Work out the finished part from the listing and answer in its coordinate system (mm). A direction names the side the tool comes from. Coordinates: 2 decimals unless noted, no trailing zeros. Order: outer loops, then holes, each group sorted by start corner. A loop starts at its lowest first (then second) coordinate and runs counter-clockwise, first axis right, second up. Notation, with made-up numbers: M 19.25,61.25 L 28.25,61.25 A21 cw 28.25,82.25 Z; hole C -5.75,-17 d3. An arc over 180 degrees is marked long. Answer in a Markdown table with one row per item. Add a question column.
Item 1: The mould has two halves that part along X. Classify faces 1 (the face through (8.5, 0.07, 78.52)), 2 (the face through (-33.89, -24.17, 21.43)), 3 (the face through (-26.45, 31, 12)): released by +X, released by -X, zero draft, split by the parting line, or undercut.
Item 2: Which of the six approach directions +Z, -Z, +X, -X, +Y, -Y give full straight-line access (tool end or side, diameter ignored) to faces 4 (the face through (26.45, -28, 17)), 5 (the face through (-33.9, 24.6, 22)), 6 (the face through (33.9, 24.6, 22))?
Item 3: The part is cut by section C-C (z = 65). Write down the section's boundary in (x, y), then the cut area to 3 significant figures.
Item 4: The part is cut by section B-B (y = 0). Write down the section's boundary in (x, z).
Item 5: Consider line 1 (Y direction, x = -10, z = 79.2); line 2 (X direction, y = -24, z = 46.5); line 3 (Z direction, x = 5.5, y = 17). Determine where each line is inside the solid, lowest interval first. Write a range as from..to.
Item 6: The part is cut by section D-D (y = 19.5). Write down the section's boundary in (x, z), then the cut area to 3 significant figures.
Item 7: A flat-ended cylindrical pin translates along its axis: pin 1 Ø4 at (x, y) = (-10, 25) entering from -Z. Find the tip coordinate at first contact, or state that the pin passes through.
Item 8: The part is cut by section A-A (x = -10). Write down the section's boundary in (y, z), then the cut area to 3 significant figures.
from build123d import *

# Parameters (mm, degrees)
SKETCH_1_W          = 52.9
SKETCH_1_H          = 81.56
EXTRUDE_1_DEPTH     = 80.99
SKETCH_2_W          = 32.9
SKETCH_2_H          = 61.56
CUT_EXTRUDE_1_DEPTH = 75.99
EXTRUDE_2_DEPTH     = 15.1
SKETCH_4_R          = 1.5
CUT_EXTRUDE_2_DEPTH = 100.743626363


with BuildPart() as part:
    # 草图1 → 凸台-拉伸1 (new body)
    with BuildSketch(Plane.XY):
        Rectangle(SKETCH_1_W, SKETCH_1_H)
    extrude(amount=EXTRUDE_1_DEPTH)

    # 草图2 → 切除-拉伸1 (cut)
    with BuildSketch(Plane(origin=(0, 0, 0), x_dir=(-1, 0, 0), z_dir=(0, 0, -1))):
        Rectangle(SKETCH_2_W, SKETCH_2_H)
    extrude(amount=-CUT_EXTRUDE_1_DEPTH, mode=Mode.SUBTRACT)

    # 草图3 → 凸台-拉伸2 (add)
    with BuildSketch(Plane.ZY.offset(26.45)):
        Polygon((80.99, 40.78), (43.47, 40.78), (0, 8.02), (0, -8.02), (43.47, -40.78), (80.99, -40.78), align=None)
    extrude_2 = extrude(amount=EXTRUDE_2_DEPTH)

    # 镜向1: 凸台-拉伸2 across plane
    add(extrude_2.mirror(Plane(origin=(0, 0, 0), x_dir=(0, 0, 1), z_dir=(1, 0, 0))))

    # 草图4 → 切除-拉伸2 (cut, through all)
    with BuildSketch(Plane.XY.offset(80.99)):
        with Locations((-10, 25)):
            Circle(SKETCH_4_R)
        with Locations((10, 25)):
            Circle(SKETCH_4_R)
        with Locations((-10, -25)):
            Circle(SKETCH_4_R)
        with Locations((10, -25)):
            Circle(SKETCH_4_R)
        with Locations((-10, 0)):
            Circle(SKETCH_4_R)
        with Locations((10, 0)):
            Circle(SKETCH_4_R)
    extrude(amount=-CUT_EXTRUDE_2_DEPTH, mode=Mode.SUBTRACT)


solid = part.part
Reply:
| question | item | result |
|---|---|---|
| 1 | face 1 | undercut |
| 1 | face 2 | zero draft |
| 1 | face 3 | released by -X |
| 2 | face 4 | -Z, +X, -Y |
| 2 | face 5 | -Z, -X, +Y |
| 2 | face 6 | -Z, +X, +Y |
| 3 | outline | M -41.55,-40.78 L 41.55,-40.78 L 41.55,40.78 L -41.55,40.78 Z; hole M -16.45,-30.78 L 16.45,-30.78 L 16.45,30.78 L -16.45,30.78 Z |
| 3 | area | 4,750 mm2 |
| 4 | outline | M -41.55,0 L -16.45,0 L -16.45,75.99 L -11.5,75.99 L -11.5,80.99 L -41.55,80.99 Z; M -8.5,75.99 L 8.5,75.99 L 8.5,80.99 L -8.5,80.99 Z; M 11.5,75.99 L 16.45,75.99 L 16.45,0 L 41.55,0 L 41.55,80.99 L 11.5,80.99 Z |
| 5 | line 1 | y = -40.78..-26.5, -23.5..-1.5, 1.5..23.5, 26.5..40.78 |
| 5 | line 2 | x = -41.55..-16.45, 16.45..41.55 |
| 5 | line 3 | z = 75.99..80.99 |
| 6 | outline | M -41.55,15.23 L -26.45,15.23 L -26.45,0 L -16.45,0 L -16.45,75.99 L 16.45,75.99 L 16.45,0 L 26.45,0 L 26.45,15.23 L 41.55,15.23 L 41.55,80.99 L -41.55,80.99 Z |
| 6 | area | 3,770 mm2 |
| 7 | pin 1 | stops at z = 75.99 |
| 8 | outline | M -40.78,0 L -30.78,0 L -30.78,75.99 L -26.5,75.99 L -26.5,80.99 L -40.78,80.99 Z; M -23.5,75.99 L -1.5,75.99 L -1.5,80.99 L -23.5,80.99 Z; M 1.5,75.99 L 23.5,75.99 L 23.5,80.99 L 1.5,80.99 Z; M 26.5,75.99 L 30.78,75.99 L 30.78,0 L 40.78,0 L 40.78,80.99 L 26.5,80.99 Z |
| 8 | area | 1,880 mm2 |
